```python
from build123d import *

# Parameters (mm, degrees)
SKETCH1_R           = 1
BOSS_EXTRUDE1_DEPTH = 2
MOVE_FACE1_BY       = 0.25
MOVE_FACE1_2_BY     = 0.25


with BuildPart() as part:
    # Sketch1 → Boss-Extrude1 (new body)
    with BuildSketch(Plane(origin=(0, 0, 0), x_dir=(1, 0, 0), z_dir=(0, 1, 0))):
        with BuildLine():
            Line((-2.5, 0), (-2.5, 18))
            ThreePointArc((-2.5, 18), (0, 20.5), (2.5, 18))
            Line((2.5, 18), (2.5, 0))
            ThreePointArc((2.5, 0), (0, -2.5), (-2.5, 0))
        make_face()
        with Locations(Location((0, 18, 0), (0, 0, 270))):
            Circle(SKETCH1_R, mode=Mode.SUBTRACT)
        with Locations(Location((0, 0, 0), (0, 0, 270))):
            Circle(SKETCH1_R, mode=Mode.SUBTRACT)
    extrude(amount=BOSS_EXTRUDE1_DEPTH)

    # Move Face1: a curved face moved inward by 0.25
    add(Solid.thicken(part.faces().sort_by_distance((0, 1, -1))[0], -MOVE_FACE1_BY), mode=Mode.SUBTRACT)

    # Move Face1 2: a curved face moved inward by 0.25
    add(Solid.thicken(part.faces().sort_by_distance((0, 1, -19))[0], -MOVE_FACE1_2_BY), mode=Mode.SUBTRACT)


solid = part.part
```
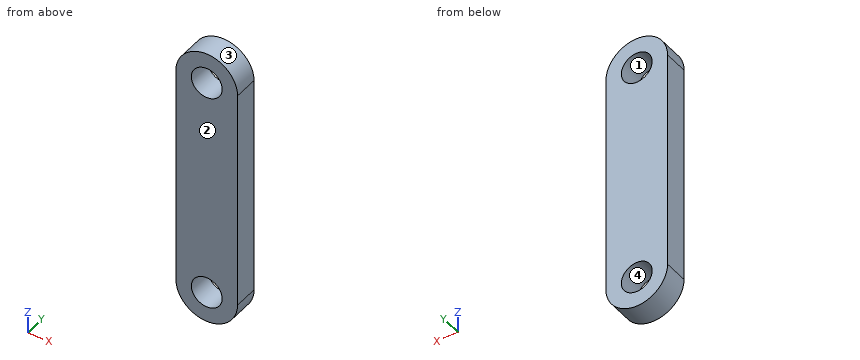
Source: CAD feature listing. Evaluate the final solid. Frame: model axes, mm. Face numbers are marked on the shaded views. Give positions to 0.01 mm unless a question says otherwise; leave off trailing zeros. Loops run counter-clockwise (first coordinate to the right, second up) from the corner with the lowest first, then second, coordinate; pieces in that order, holes last. Notation, with made-up numbers: (-36, 49) - (23, 49) arc R12 cw to (23, 53) - close; hole circle Ø2 at (-1.75, -18.75). An arc over 180 degrees is marked (long way). Use CSV: the item, a comma, the result in double quotes.
1) Cut plane C-C (x = 2.15). Output: boundary loops of the cut face in (y, z), and give its area (3 significant figures).
Worked out:
outline,"(0, -19.28) - (2, -19.28) - (2, 1.28) - (0, 1.28) - close"
area,"41.1 mm^2"
2) Cut plane B-B (x = -0.95). Output: boundary loops of the cut face in (y, z), and give its area (3 significant figures).
Worked out:
outline,"(0, -20.31) - (2, -20.31) - (2, -18.81) - (0, -18.81) - close; (0, -17.19) - (2, -17.19) - (2, -0.81) - (0, -0.81) - close; (0, 0.81) - (2, 0.81) - (2, 2.31) - (0, 2.31) - close"
area,"38.8 mm^2"
3) Mould query, pull axis X, two halves, no side actions, for the marked faces 1, 2, 3 and 4. Classes: +X half, -X half, draft (parallel to the pull), parting line (faces both ways), or undercut.
Worked out:
face 1,"undercut"
face 2,"draft"
face 3,"parting line"
face 4,"undercut"
4) Pin query (flat end, axial travel): P1, Ø3, axis at x = 0, z = -18, coming from the -Y side. Return the tip coordinate at first contact, or that it passes through.
Worked out:
P1,"stops at y = 0"
5) Cut plane A-A (x = 0). Output: boundary loops of the cut face in (y, z), and give its area (3 significant figures).
Worked out:
outline,"(0, -20.5) - (2, -20.5) - (2, -19.25) - (0, -19.25) - close; (0, -16.75) - (2, -16.75) - (2, -1.25) - (0, -1.25) - close; (0, 1.25) - (2, 1.25) - (2, 2.5) - (0, 2.5) - close"
area,"36.0 mm^2"
6) Line query: line 1 (Z direction, x = 0.6, y = 1.05); line 2 (Z direction, x = 1, y = 0.2); line 3 (X direction, y = 1.3, z = -18). Output: solid intervals per line, ascending.
Worked out:
line 1,"z = -20.43 to -19.1, -16.9 to -1.1, 1.1 to 2.43"
line 2,"z = -20.29 to -18.75, -17.25 to -0.75, 0.75 to 2.29"
line 3,"x = -2.5 to -1.25, 1.25 to 2.5"
